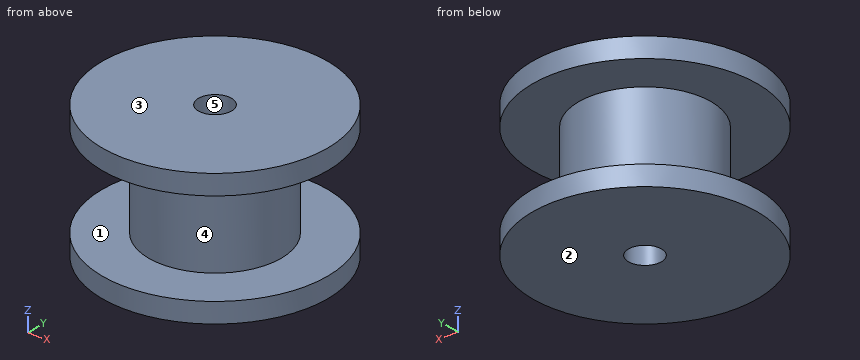
```python
from build123d import *

# Parameters (mm, degrees)
TALADRO_ROSCADO_M2_52_D = 2.5


with BuildPart() as part:
    # Sketch2 → Revolve1 (revolve)
    with BuildSketch(Plane(origin=(0, 0, 0), x_dir=(1, 0, 0), z_dir=(0, 1, 0)), mode=Mode.PRIVATE) as revolve1_sk:
        Polygon((0, 10), (-8.5, 10), (-8.5, 8.5), (-5, 8.5), (-5, 1.5), (-8.5, 1.5), (-8.5, 0), (0, 0), align=None)
    revolve(revolve1_sk.sketch.rotate(Axis((0, 0, 198.467795094), (0, 0, -1)), 180), axis=Axis((0, 0, 198.467795094), (0, 0, -1)))

    # Taladro roscado M2.52 (through all)
    with Locations(Plane.XY):
        with Locations((0, 0)):
            Hole(TALADRO_ROSCADO_M2_52_D / 2)


solid = part.part
```
Here's how the part is built. I have some questions about the finished solid (model axes, mm). Face numbers are marked on the shaded views. A direction names the side the tool comes from. Coordinates: 2 decimals unless noted, no trailing zeros. Order: outer loops, then holes, each group sorted by start corner. A loop starts at its lowest first (then second) coordinate and runs counter-clockwise, first axis right, second up. Notation, with made-up numbers: (60, -36.75) - (69, -36.75) arc R18 cw to (69, -30.75) - close; hole circle Ø10 at (32, 3). An arc over 180 degrees is marked (long way). One line per question, with ' | ' between items. Start each with the question number.
1. If we section it at C-C (z = -9): Write out the boundary of the cut face in (x, y).
2. Which directions (+Z, -Z, +X, -X, +Y, -Y) give clear straight access to the entire face, cutting with the end or side of a thin tool? Please do the marked faces 4 and 5.
3. If we section it at D-D (x = 3.5): Write out the boundary of the cut face in (y, z).
4. I'm going to push flat-ended pins straight in: pin 1 Ø3 at (x, z) = (-2.5, -3.5) entering from -Y; pin 2 Ø1.5 at (x, z) = (-2, -6) entering from -Y; pin 3 Ø1.5 at (y, z) = (4, -2.5) entering from -X; pin 4 Ø2 at (x, y) = (0, 0) entering from +Z. Where does each tip first touch, or does it pass through?
5. Please list where these lines run through material, in increasing order: line 1 along Y through (x, z) = (0, -6); line 2 along Z through (x, y) = (-4.5, 4.5); line 3 along Y through (x, z) = (-0.5, -4.75). Write a range as [from, to].
6. If we section it at A-A (y = -5.75): Write out the boundary of the cut face in (x, z).
7. If we section it at B-B (x = 0): Write out the boundary of the cut face in (y, z).
8. If we mould it in two halves opening along Z, with no side actions, what happens to the marked faces 1, 2 and 3? For each: released by +Z, released by -Z, zero draft, split by the parting line, or undercut.
Model answer:
1) outline: circle Ø17 at (0, 0); hole circle Ø2.5 at (0, 0)
2) face 4: none | face 5: +Z, -Z
3) outline: (-7.75, -10) - (7.75, -10) - (7.75, -8.5) - (3.57, -8.5) - (3.57, -1.5) - (7.75, -1.5) - (7.75, 0) - (-7.75, 0) - (-7.75, -1.5) - (-3.57, -1.5) - (-3.57, -8.5) - (-7.75, -8.5) - close
4) pin 1: stops at y = -4.9 | pin 2: stops at y = -4.84 | pin 3: stops at x = -3.8 | pin 4: passes through
5) line 1: y = [-5, -1.25], [1.25, 5] | line 2: z = [-10, -8.5], [-1.5, 0] | line 3: y = [-4.97, -1.15], [1.15, 4.97]
6) outline: (-6.26, -10) - (6.26, -10) - (6.26, -8.5) - (-6.26, -8.5) - close; (-6.26, -1.5) - (6.26, -1.5) - (6.26, 0) - (-6.26, 0) - close
7) outline: (-8.5, -10) - (-1.25, -10) - (-1.25, 0) - (-8.5, 0) - (-8.5, -1.5) - (-5, -1.5) - (-5, -8.5) - (-8.5, -8.5) - close; (1.25, -10) - (8.5, -10) - (8.5, -8.5) - (5, -8.5) - (5, -1.5) - (8.5, -1.5) - (8.5, 0) - (1.25, 0) - close
8) face 1: undercut | face 2: released by -Z | face 3: released by +Z
